The listing builds one solid part. Answer for the finished solid, in the listing's coordinates (mm). A direction names the side the tool comes from. Give positions to 0.01 mm unless a question says otherwise; leave off trailing zeros. Order: outer loops, then holes, each group sorted by start corner. A loop starts at its lowest first (then second) coordinate and runs counter-clockwise, first axis right, second up. Notation, with made-up numbers: (27, -14) - (58, -14) arc R23 ccw to (58, 17) - close; hole circle Ø3 at (86, 34.5). An arc over 180 degrees is marked (long way). Use a Markdown table: item, result. Add a question column.
1) Straight lines are drawn through the part: line 1 (Y direction, x = 9, z = 0); line 2 (Y direction, x = 8.25, z = -0.5); line 3 (X direction, y = 5, z = -3.5). For each, find the intervals that lie inside material, in ascending order.
2) The mould has two halves that part along Z. Classify faces 1 (the face through (0, -1.5, -0.1)), 2 (the face through (9.94, -0.54, -12.19)), 3 (the face through (18, -1.5, 0.1)): released by +Z, released by -Z, zero draft, split by the parting line, or undercut.
3) Find section A-A, the plane z = 0. Determine the outline of the cut face in (x, y), plus the area to 3 significant figures.
4) Flat-ended cylindrical pins translate along their axes: pin 1 (8 mm diameter, centred on x = 11.5, z = 7, fed in from +Y); pin 2 (3 mm diameter, centred on y = 0, z = 0, fed in from +X); pin 3 (3 mm diameter, centred on x = 6.5, z = -9, fed in from -Y). Find the tip coordinate at first contact, or state that the pin passes through.
5) For faces 4 (the face through (18.8, -1.9, 5.9)), 5 (the face through (9.13, -1.01, 0.65)), determine the directions among +Z, -Z, +X, -X, +Y, -Y from which every point of the face is accessible in a straight line to the end or side of a thin tool.
from build123d import *


with BuildPart() as part:
    # Sketch1 → Revolve1 (revolve)
    with BuildSketch(Plane(origin=(0, 0, 0), x_dir=(1, 0, 0), z_dir=(0, 1, 0)), mode=Mode.PRIVATE) as revolve1_sk:
        with BuildLine():
            Line((19.5, 6.2), (19.980711996, 6.680711996))
            ThreePointArc((19.980711996, 6.680711996), (18.069135536, 10.609323756), (14, 12.2))
            Line((14, 12.2), (6, 12.2))
            ThreePointArc((6, 12.2), (1.757359313, 10.442640687), (0, 6.2))
            Line((0, 6.2), (0, 1.2))
            Line((0, 1.2), (18, 1.2))
            Line((18, 1.2), (18, 6.2))
            Line((18, 6.2), (19.5, 6.2))
        make_face()
    revolve(revolve1_sk.sketch.rotate(Axis((0, 0, 0), (1, 0, 0)), 180), axis=Axis((0, 0, 0), (1, 0, 0)))


solid = part.part
The answers:
| question | item | result |
|---|---|---|
| 1 | line 1 | -12.2 to -1.2, 1.2 to 12.2 |
| 1 | line 2 | -12.19 to -1.09, 1.09 to 12.19 |
| 1 | line 3 | 0 to 18 |
| 2 | face 1 | zero draft |
| 2 | face 2 | split by the parting line |
| 2 | face 3 | undercut |
| 3 | outline | (0, -6.2) arc R6 ccw to (6, -12.2) - (14, -12.2) arc R6 ccw to (19.98, -6.68) - (19.5, -6.2) - (18, -6.2) - (18, -1.2) - (0, -1.2) - close; (0, 1.2) - (18, 1.2) - (18, 6.2) - (19.5, 6.2) - (19.98, 6.68) arc R6 ccw to (14, 12.2) - (6, 12.2) arc R6 ccw to (0, 6.2) - close |
| 3 | area | 389 mm2 |
| 4 | pin 1 | y = 11.83 |
| 4 | pin 2 | x = 18 |
| 4 | pin 3 | y = -9.62 |
| 5 | face 4 | +X |
| 5 | face 5 | +X, -X |
